Part model, mm, in its own coordinate system. A direction names the side the tool comes from. Round coordinates to 2 decimals unless told otherwise and drop trailing zeros. Write each loop counter-clockwise with the first axis right and the second up, starting at its lowest first coordinate (ties: lowest second). Pieces come first, ordered by that corner, then holes.
```python
from build123d import *
from build123d.topology import SkipClean

# Parameters (mm, degrees)
SKETCH2_R           = 25
BOSS_EXTRUDE1_DEPTH = 14.6
BOSS_EXTRUDE2_START = 40
SKETCH3_R           = 46.5
SKETCH3_R_2         = 25
BOSS_EXTRUDE2_DEPTH = 40
SKETCH6_W           = 12
SKETCH6_H           = 17.793467461
CUT_EXTRUDE1_DEPTH  = 64
CHAMFER1_SIZE       = 1.5
CHAMFER2_SIZE       = 8


with BuildPart() as part:
    # Sketch2 → Boss-Extrude1 (new body)
    with BuildSketch(Plane.XY):
        with BuildLine():
            ThreePointArc((-52.801936247, 70.154195014), (-51.720450563, 65.277064388), (-50.066512977, 60.563201335))
            ThreePointArc((-50.066512977, 60.563201335), (-51.791439328, 51.791439328), (-60.563201335, 50.066512977))
            ThreePointArc((-60.563201335, 50.066512977), (-65.277064388, 51.720450563), (-70.154195014, 52.801936247))
            ThreePointArc((-70.154195014, 52.801936247), (-71.035449372, 51.610274965), (-71.896464027, 50.403908677))
            ThreePointArc((-71.896464027, 50.403908677), (-69.360793773, 46.09967927), (-66.331141862, 42.127623919))
            ThreePointArc((-66.331141862, 42.127623919), (-65.261020777, 33.252150946), (-73.070430637, 28.901024969))
            ThreePointArc((-73.070430637, 28.901024969), (-78.064675632, 29.017349295), (-83.03729995, 28.538787055))
            ThreePointArc((-83.03729995, 28.538787055), (-83.507179062, 27.133127254), (-83.953264975, 25.719736574))
            ThreePointArc((-83.953264975, 25.719736574), (-80.211619223, 22.40973635), (-76.102816424, 19.568301152))
            ThreePointArc((-76.102816424, 19.568301152), (-72.342398812, 11.457910348), (-78.425017076, 4.906503271))
            ThreePointArc((-78.425017076, 4.906503271), (-83.210772516, 3.473827702), (-87.792135411, 1.482062544))
            ThreePointArc((-87.792135411, 1.482062544), (-87.804644236, 0), (-87.792135411, -1.482062544))
            ThreePointArc((-87.792135411, -1.482062544), (-83.210772516, -3.473827702), (-78.425017076, -4.906503271))
            ThreePointArc((-78.425017076, -4.906503271), (-72.342398812, -11.457910348), (-76.102816424, -19.568301152))
            ThreePointArc((-76.102816424, -19.568301152), (-80.211619223, -22.40973635), (-83.953264975, -25.719736574))
            ThreePointArc((-83.953264975, -25.719736574), (-83.507179062, -27.133127254), (-83.03729995, -28.538787055))
            ThreePointArc((-83.03729995, -28.538787055), (-78.064675632, -29.017349295), (-73.070430637, -28.901024969))
            ThreePointArc((-73.070430637, -28.901024969), (-65.261020777, -33.252150946), (-66.331141862, -42.127623918))
            ThreePointArc((-66.331141862, -42.127623918), (-69.360793773, -46.09967927), (-71.896464027, -50.403908677))
            ThreePointArc((-71.896464027, -50.403908677), (-71.035449372, -51.610274965), (-70.154195014, -52.801936247))
            ThreePointArc((-70.154195014, -52.801936247), (-65.277064388, -51.720450563), (-60.563201335, -50.066512977))
            ThreePointArc((-60.563201335, -50.066512977), (-51.791439328, -51.791439328), (-50.066512977, -60.563201335))
            ThreePointArc((-50.066512977, -60.563201335), (-51.720450563, -65.277064388), (-52.801936247, -70.154195014))
            ThreePointArc((-52.801936247, -70.154195014), (-51.610274965, -71.035449372), (-50.403908677, -71.896464027))
            ThreePointArc((-50.403908677, -71.896464027), (-46.09967927, -69.360793773), (-42.127623918, -66.331141861))
            ThreePointArc((-42.127623918, -66.331141861), (-33.252150946, -65.261020777), (-28.901024969, -73.070430637))
            ThreePointArc((-28.901024969, -73.070430637), (-29.017349295, -78.064675632), (-28.538787055, -83.03729995))
            ThreePointArc((-28.538787055, -83.03729995), (-27.133127254, -83.507179062), (-25.719736574, -83.953264975))
            ThreePointArc((-25.719736574, -83.953264975), (-22.40973635, -80.211619223), (-19.568301152, -76.102816424))
            ThreePointArc((-19.568301152, -76.102816424), (-11.457910348, -72.342398812), (-4.906503271, -78.425017076))
            ThreePointArc((-4.906503271, -78.425017076), (-3.473827702, -83.210772516), (-1.482062544, -87.792135411))
            ThreePointArc((-1.482062544, -87.792135411), (0, -87.804644236), (1.482062544, -87.792135411))
            ThreePointArc((1.482062544, -87.792135411), (3.473827702, -83.210772516), (4.906503271, -78.425017076))
            ThreePointArc((4.906503271, -78.425017076), (11.457910348, -72.342398812), (19.568301152, -76.102816424))
            ThreePointArc((19.568301152, -76.102816424), (22.40973635, -80.211619223), (25.719736574, -83.953264975))
            ThreePointArc((25.719736574, -83.953264975), (27.133127254, -83.507179062), (28.538787055, -83.03729995))
            ThreePointArc((28.538787055, -83.03729995), (29.017349295, -78.064675632), (28.901024969, -73.070430637))
            ThreePointArc((28.901024969, -73.070430637), (33.252150946, -65.261020777), (42.127623918, -66.331141861))
            ThreePointArc((42.127623918, -66.331141861), (46.09967927, -69.360793773), (50.403908677, -71.896464027))
            ThreePointArc((50.403908677, -71.896464027), (51.610274965, -71.035449372), (52.801936247, -70.154195014))
            ThreePointArc((52.801936247, -70.154195014), (51.720450563, -65.277064388), (50.066512977, -60.563201335))
            ThreePointArc((50.066512977, -60.563201335), (51.791439328, -51.791439328), (60.563201335, -50.066512977))
            ThreePointArc((60.563201335, -50.066512977), (65.277064388, -51.720450563), (70.154195014, -52.801936247))
            ThreePointArc((70.154195014, -52.801936247), (71.035449372, -51.610274965), (71.896464027, -50.403908677))
            ThreePointArc((71.896464027, -50.403908677), (69.360793773, -46.09967927), (66.331141862, -42.127623919))
            ThreePointArc((66.331141862, -42.127623919), (65.261020777, -33.252150946), (73.070430637, -28.901024969))
            ThreePointArc((73.070430637, -28.901024969), (78.064675632, -29.017349295), (83.03729995, -28.538787055))
            ThreePointArc((83.03729995, -28.538787055), (83.507179062, -27.133127254), (83.953264975, -25.719736574))
            ThreePointArc((83.953264975, -25.719736574), (80.211619223, -22.40973635), (76.102816424, -19.568301152))
            ThreePointArc((76.102816424, -19.568301152), (72.342398812, -11.457910348), (78.425017076, -4.906503271))
            ThreePointArc((78.425017076, -4.906503271), (83.210772516, -3.473827702), (87.792135411, -1.482062544))
            ThreePointArc((87.792135411, -1.482062544), (87.804644236, 0), (87.792135411, 1.482062544))
            ThreePointArc((87.792135411, 1.482062544), (83.210772516, 3.473827702), (78.425017076, 4.906503271))
            ThreePointArc((78.425017076, 4.906503271), (72.342398812, 11.457910348), (76.102816424, 19.568301152))
            ThreePointArc((76.102816424, 19.568301152), (80.211619223, 22.40973635), (83.953264975, 25.719736575))
            ThreePointArc((83.953264975, 25.719736575), (83.507179062, 27.133127254), (83.03729995, 28.538787055))
            ThreePointArc((83.03729995, 28.538787055), (78.064675632, 29.017349295), (73.070430637, 28.901024969))
            ThreePointArc((73.070430637, 28.901024969), (65.261020777, 33.252150946), (66.331141862, 42.127623918))
            ThreePointArc((66.331141862, 42.127623918), (69.360793773, 46.09967927), (71.896464027, 50.403908677))
            ThreePointArc((71.896464027, 50.403908677), (71.035449372, 51.610274965), (70.154195014, 52.801936247))
            ThreePointArc((70.154195014, 52.801936247), (65.277064388, 51.720450563), (60.563201335, 50.066512977))
            ThreePointArc((60.563201335, 50.066512977), (51.791439328, 51.791439328), (50.066512977, 60.563201335))
            ThreePointArc((50.066512977, 60.563201335), (51.720450563, 65.277064388), (52.801936247, 70.154195014))
            ThreePointArc((52.801936247, 70.154195014), (51.610274965, 71.035449372), (50.403908677, 71.896464027))
            ThreePointArc((50.403908677, 71.896464027), (46.09967927, 69.360793773), (42.127623918, 66.331141861))
            ThreePointArc((42.127623918, 66.331141861), (33.252150946, 65.261020777), (28.901024969, 73.070430637))
            ThreePointArc((28.901024969, 73.070430637), (29.017349295, 78.064675632), (28.538787055, 83.03729995))
            ThreePointArc((28.538787055, 83.03729995), (27.133127254, 83.507179062), (25.719736574, 83.953264975))
            ThreePointArc((25.719736574, 83.953264975), (22.40973635, 80.211619223), (19.568301152, 76.102816424))
            ThreePointArc((19.568301152, 76.102816424), (11.457910348, 72.342398812), (4.906503271, 78.425017076))
            ThreePointArc((4.906503271, 78.425017076), (3.473827702, 83.210772516), (1.482062544, 87.792135411))
            ThreePointArc((1.482062544, 87.792135411), (0, 87.804644236), (-1.482062544, 87.792135411))
            ThreePointArc((-1.482062544, 87.792135411), (-3.473827702, 83.210772516), (-4.906503271, 78.425017076))
            ThreePointArc((-4.906503271, 78.425017076), (-11.457910348, 72.342398812), (-19.568301152, 76.102816424))
            ThreePointArc((-19.568301152, 76.102816424), (-22.40973635, 80.211619223), (-25.719736574, 83.953264975))
            ThreePointArc((-25.719736574, 83.953264975), (-27.133127254, 83.507179062), (-28.538787055, 83.03729995))
            ThreePointArc((-28.538787055, 83.03729995), (-29.017349295, 78.064675632), (-28.901024969, 73.070430637))
            ThreePointArc((-28.901024969, 73.070430637), (-33.252150946, 65.261020777), (-42.127623918, 66.331141862))
            ThreePointArc((-42.127623918, 66.331141862), (-46.09967927, 69.360793773), (-50.403908677, 71.896464027))
            ThreePointArc((-50.403908677, 71.896464027), (-51.610274965, 71.035449372), (-52.801936247, 70.154195014))
        make_face()
        Circle(SKETCH2_R, mode=Mode.SUBTRACT)
    extrude(amount=BOSS_EXTRUDE1_DEPTH)

    # Sketch3 → Boss-Extrude2 (add)
    with SkipClean():  # the faces are left unmerged after this step: merging them gives an invalid solid
        with BuildSketch(Plane(origin=(0, 0, 14.6), x_dir=(-1, 0, 0), z_dir=(0, 0, -1)).offset(BOSS_EXTRUDE2_START)):
            with Locations(Location((0, 0, 0), (0, 0, 180))):
                Circle(SKETCH3_R)
            Circle(SKETCH3_R_2, mode=Mode.SUBTRACT)
        extrude(amount=-BOSS_EXTRUDE2_DEPTH)

    # Sketch6 → Cut-Extrude1 (cut)
    with SkipClean():  # the faces are left unmerged after this step: merging them gives an invalid solid
        with BuildSketch(Plane(origin=(0, 0, -25.4), x_dir=(-1, 0, 0), z_dir=(0, 0, -1))):
            with Locations((0, 20.10326627)):
                Rectangle(SKETCH6_W, SKETCH6_H)
        extrude(amount=-CUT_EXTRUDE1_DEPTH, mode=Mode.SUBTRACT)
    add(part.part.scale(1), mode=Mode.REPLACE)  # the faces are merged on a copy

    # Chamfer1
    chamfer1_edges = [part.edges().sort_by_distance(p)[0] for p in [
        (-46.5, 0, -25.4),
        (15.411035007, -19.685019685, -25.4),
        (-6, 26.6346611, -25.4),
        (6, 26.6346611, -25.4),
        (-15.411035007, -19.685019685, 14.6),
        (0, 29, -25.4),
    ]]
    chamfer(chamfer1_edges, length=CHAMFER1_SIZE)

    # Chamfer2
    chamfer2_edges = [part.edges().sort_by_distance(p)[0] for p in [
        (-46.5, 0, 0),
    ]]
    chamfer(chamfer2_edges, length=CHAMFER2_SIZE)


solid = part.part
```
Q1. Wall check: L1, parallel to Y at x = 0, z = -12; L2, parallel to Y at x = 28.5, z = 12; L3, parallel to Z at x = -68, y = -13. Give the ranges that are in metal, low to high.
Values follow:
L1: y = -46.5 to -25, 29 to 46.5
L2: y = -83.05 to 83.05
L3: z = 0 to 14.6
Q2. Cut at A-A on z = -12. Write the cut outline in (x, y), plus the area to 3 significant figures.
Values follow:
outline: circle Ø93 at (0, 0); hole (-6, 24.27) arc R25 ccw (long way) to (6, 24.27) - (6, 29) - (-6, 29) - close
area: 4,780 mm2
Q3. Which spindle directions (+Z, -Z, +X, -X, +Y, -Y) get a long thin tool onto all of the face, cutting with end or side? Do faces 4 (the cylindrical face through (-80.267, 22.453, 7.198)), 5 (the cylindrical face through (44.35, -13.97, -16.06)), 6 (the flat face through (0, 29, -5)). Say none if no direction does.
Values follow:
face 4: +Z, -Z, -X
face 5: -Z
face 6: +Z, -Z
Q4. Drop flat-ended pins along their axis: pin 1 (6 mm diameter, centred on x = 0.5, z = -9, fed in from -Y); pin 2 (5 mm diameter, centred on x = -23.5, y = -5.5, fed in from -Z); pin 3 (5 mm diameter, centred on y = 26.5, z = -7.5, fed in from -X); pin 4 (5 mm diameter, centred on y = 26.5, z = -13, fed in from +X). Give the stop position or say it passes through.
Values follow:
pin 1: stops at y = -48.5
pin 2: stops at z = -25.4
pin 3: stops at x = -42.19
pin 4: stops at x = 39.83
Q5. Mould opens along X. For faces 1 (the cylindrical face through (-51.7, -65.2, 7.2)), 2 (the cylindrical face through (-51.886, -51.698, 7.198)), 3 (the cylindrical face through (51.7, 65.2, 7.2)) say: +X half, -X half, draft (parallel to the pull), parting line (faces both ways), or undercut.
Values follow:
face 1: -X half
face 2: undercut
face 3: +X half
